Can you work these out from the model? Positions are in its coordinate system, mm. Face numbers are marked on the shaded views. Give positions to 0.01 mm unless a question says otherwise; leave off trailing zeros. Order: outer loops, then holes, each group sorted by start corner. A loop starts at its lowest first (then second) coordinate and runs counter-clockwise, first axis right, second up. Notation, with made-up numbers: (-25, 26) - (24, 26) arc R19 ccw to (24, 31) - close; hole circle Ø9 at (71, 76.5). An arc over 180 degrees is marked (long way). One line per question, with ' | ' between items.
```python
from build123d import *

# Parameters (mm, degrees)
F0_W     = 76.2
F0_H     = 38.1
F0_W_2   = 4.3388303002
F0_H_2   = 20.4583236755
F1_DEPTH = 12.7


with BuildPart() as f1:
    # F0 (on Top) → F1 (new body)
    with BuildSketch(Plane.XY):
        Rectangle(F0_W, F0_H)
        with BuildLine():
            Line((-24.7102881895, -1.7794135219), (-27.0162712695, -1.7794135219))
            Line((-27.0162712695, -1.7794135219), (-27.0162712695, -9.6287112683))
            Line((-27.0162712695, -9.6287112683), (-31.3551015697, -9.6287112683))
            Line((-31.3551015697, -9.6287112683), (-31.3551015697, 10.8296124072))
            Line((-31.3551015697, 10.8296124072), (-25.3953666579, 10.8296124072))
            add(Edge.make_bspline(
                [(-25.3953666579, 10.8296124072), (-21.2222089285, 10.8296124072), (-19.2229439863, 9.3116934477)],
                knots=[0, 0, 0, 1, 1, 1], degree=2))
            add(Edge.make_bspline(
                [(-19.2229439863, 9.3116934477), (-17.223679044, 7.7937744882), (-17.223679044, 4.6997272875)],
                knots=[0, 0, 0, 1, 1, 1], degree=2))
            add(Edge.make_bspline(
                [(-17.223679044, 4.6997272875), (-17.223679044, 2.8952395569), (-18.2154756503, 1.4892615236)],
                knots=[0, 0, 0, 1, 1, 1], degree=2))
            add(Edge.make_bspline(
                [(-18.2154756503, 1.4892615236), (-19.2072722566, 0.0832834903), (-21.0296705354, -0.7137359044)],
                knots=[0, 0, 0, 1, 1, 1], degree=2))
            add(Edge.make_bspline(
                [(-21.0296705354, -0.7137359044), (-16.4087491012, -7.6137745964), (-15.011726342, -9.6287112683)],
                knots=[0, 0, 0, 1, 1, 1], degree=2))
            Line((-15.011726342, -9.6287112683), (-19.8251861693, -9.6287112683))
            Line((-19.8251861693, -9.6287112683), (-24.7102881895, -1.7794135219))
        make_face(mode=Mode.SUBTRACT)
        with Locations((-10.2676698889, 0.6004505694)):
            Rectangle(F0_W_2, F0_H_2, mode=Mode.SUBTRACT)
        with BuildLine():
            add(Edge.make_bspline(
                [(8.0212386365, 7.1064572012), (6.8615306409, 7.5116833541), (5.7421213787, 7.5116833541)],
                knots=[0, 0, 0, 1, 1, 1], degree=2))
            add(Edge.make_bspline(
                [(5.7421213787, 7.5116833541), (3.2928539131, 7.5116833541), (1.9495627985, 5.6713745271)],
                knots=[0, 0, 0, 1, 1, 1], degree=2))
            add(Edge.make_bspline(
                [(1.9495627985, 5.6713745271), (0.6062716839, 3.8310657001), (0.6062716839, 0.5444801063)],
                knots=[0, 0, 0, 1, 1, 1], degree=2))
            add(Edge.make_bspline(
                [(0.6062716839, 0.5444801063), (0.6062716839, -6.2973493041), (5.7421213787, -6.2973493041)],
                knots=[0, 0, 0, 1, 1, 1], degree=2))
            add(Edge.make_bspline(
                [(5.7421213787, -6.2973493041), (7.8958647991, -6.2973493041), (10.9585685404, -5.2227164124)],
                knots=[0, 0, 0, 1, 1, 1], degree=2))
            Line((10.9585685404, -5.2227164124), (10.9585685404, -8.8585576959))
            add(Edge.make_bspline(
                [(10.9585685404, -8.8585576959), (8.4421365191, -9.9108024024), (5.3346564073, -9.9108024024)],
                knots=[0, 0, 0, 1, 1, 1], degree=2))
            add(Edge.make_bspline(
                [(5.3346564073, -9.9108024024), (0.8704522697, -9.9108024024), (-1.493740092, -7.2018319879)],
                knots=[0, 0, 0, 1, 1, 1], degree=2))
            add(Edge.make_bspline(
                [(-1.493740092, -7.2018319879), (-3.8579324537, -4.4928615735), (-3.8579324537, 0.5713459286)],
                knots=[0, 0, 0, 1, 1, 1], degree=2))
            add(Edge.make_bspline(
                [(-3.8579324537, 0.5713459286), (-3.8579324537, 3.7639011443), (-2.6959856395, 6.1639146024)],
                knots=[0, 0, 0, 1, 1, 1], degree=2))
            add(Edge.make_bspline(
                [(-2.6959856395, 6.1639146024), (-1.5340388254, 8.5639280605), (0.6420927803, 9.8422934379)],
                knots=[0, 0, 0, 1, 1, 1], degree=2))
            add(Edge.make_bspline(
                [(0.6420927803, 9.8422934379), (2.8182243859, 11.1206588153), (5.7421213787, 11.1206588153)],
                knots=[0, 0, 0, 1, 1, 1], degree=2))
            add(Edge.make_bspline(
                [(5.7421213787, 11.1206588153), (8.7197500161, 11.1206588153), (11.7287221128, 9.6833373227)],
                knots=[0, 0, 0, 1, 1, 1], degree=2))
            Line((11.7287221128, 9.6833373227), (10.3316993536, 6.1549593283))
            add(Edge.make_bspline(
                [(10.3316993536, 6.1549593283), (9.1809466321, 6.7012310483), (8.0212386365, 7.1064572012)],
                knots=[0, 0, 0, 1, 1, 1], degree=2))
        make_face(mode=Mode.SUBTRACT)
        Polygon((32.0751048621, 10.8296124072), (32.0751048621, -9.6287112683), (27.749707473, -9.6287112683), (27.749707473, -0.7988110083), (19.649662052, -0.7988110083), (19.649662052, -9.6287112683), (15.3108317518, -9.6287112683), (15.3108317518, 10.8296124072), (19.649662052, 10.8296124072), (19.649662052, 2.810164453), (27.749707473, 2.810164453), (27.749707473, 10.8296124072), align=None, mode=Mode.SUBTRACT)
    extrude(amount=F1_DEPTH)


solid = f1.part
```
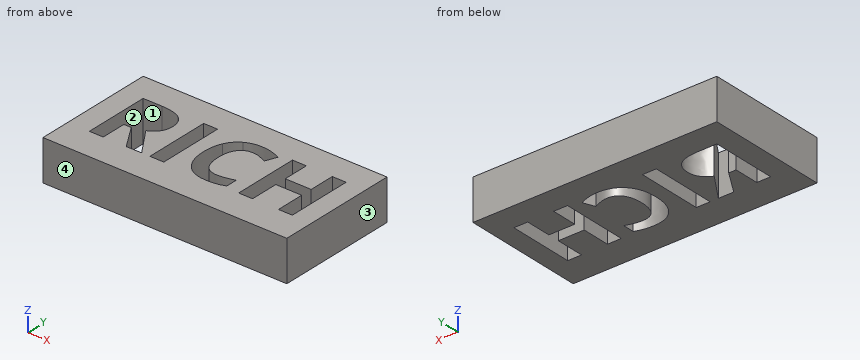
(1) Imagine slicing it at A-A (x = 24.5). List the corners of the cut face in (y, z) for me.
Answer below:
outline: (-19.05, 0) - (-0.8, 0) - (-0.8, 12.7) - (-19.05, 12.7) - close; (2.81, 0) - (19.05, 0) - (19.05, 12.7) - (2.81, 12.7) - close
(2) If we mould it in two halves opening along X, with no side actions, what happens to the marked faces 1, 2, 3 and 4? For each: released by +X, released by -X, zero draft, split by the parting line, or undercut.
Answer below:
face 1: undercut | face 2: undercut | face 3: released by +X | face 4: zero draft
(3) Imagine slicing it at B-B (z = 11.75). Count the separate pieces of the cut face and the enclosed holes in it, and give its area (3 significant figures).
Answer below:
separate pieces: 1 | enclosed holes: 4 | area: 2,230 mm^2
(4) Will this pin go through, and if not, where does the flat tip stop? pin 1 (1 mm diameter, centred on x = 6, y = -9, fed in from +Z).
Answer below:
pin 1: through
(5) If I drill on line 1 (Y direction, x = 5.5, z = 3.5); line 2 (Y direction, x = 27, z = 3); line 3 (Y direction, x = 29, z = 2.25), over which ranges is the centre line in solid material (lowest first)?
Answer below:
line 1: -19.05 to -9.91, -6.29 to 7.51, 11.12 to 19.05 | line 2: -19.05 to -0.8, 2.81 to 19.05 | line 3: -19.05 to -9.63, 10.83 to 19.05
